Job drawing, mm, ordinate dimensions from the low corner. One solid piece. A direction names the side the tool comes from. Give positions to 0.01 mm unless a question says otherwise; leave off trailing zeros. Loops run counter-clockwise (first coordinate to the right, second up) from the corner with the lowest first, then second, coordinate; pieces in that order, holes last. Notation, with made-up numbers: (-2.5, 62.5) - (10.5, 62.5) arc R24 ccw to (10.5, 93.5) - close; hole circle Ø7 at (-27, 71). An arc over 180 degrees is marked (long way). Use a Markdown table: item, result.
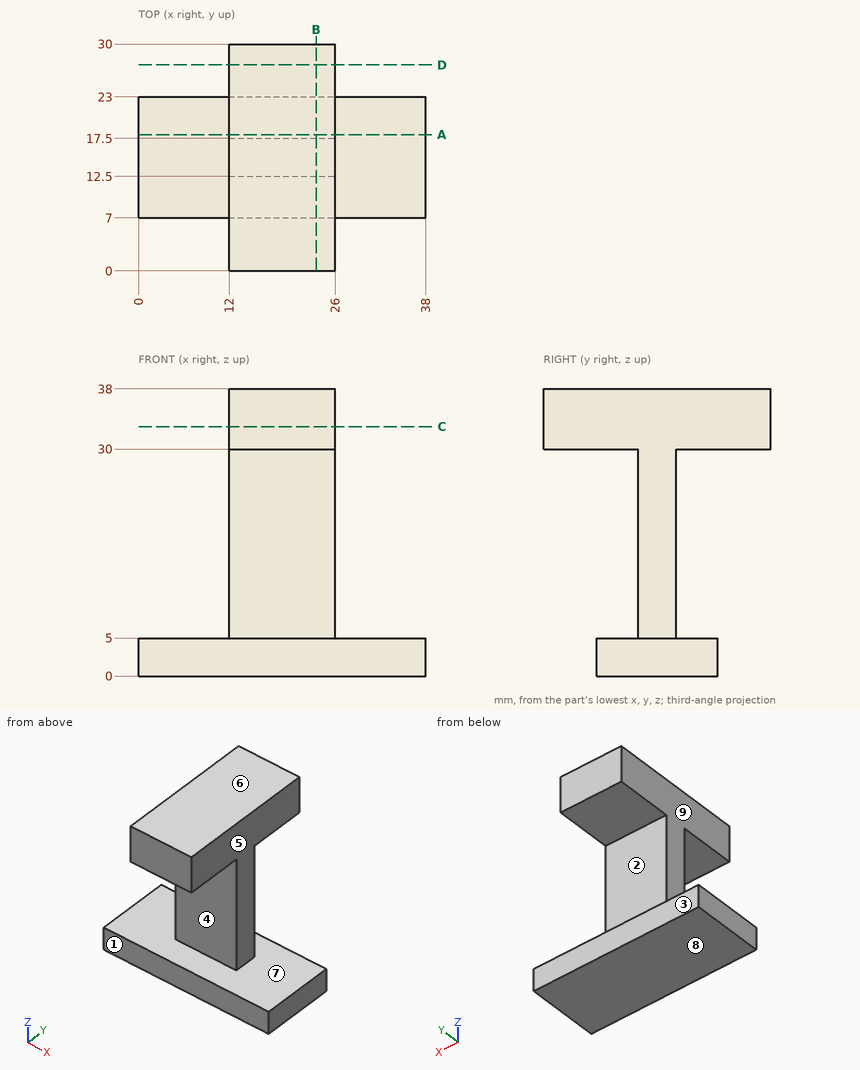
(1) Slice it at B-B, the plane x = 23.5. Write the cut outline in (y, z).
Computed:
| item | result |
|---|---|
| outline | (0, 30) - (12.5, 30) - (12.5, 5) - (7, 5) - (7, 0) - (23, 0) - (23, 5) - (17.5, 5) - (17.5, 30) - (30, 30) - (30, 38) - (0, 38) - close |
(2) Drill centre lines: probe 1 along Z at (x, y) = (7.5, 16.5); probe 2 along Y at (x, z) = (29, 4); probe 3 along Z at (x, y) = (25.5, 2.5). Where is each one in solid material? Low to high. Write a range as [from, to].
Computed:
| item | result |
|---|---|
| probe 1 | [0, 5] |
| probe 2 | [7, 23] |
| probe 3 | [30, 38] |
(3) 3-axis set-ups, long thin cutter, end or side, ignore diameter. For the marked faces 1, 2, 3, 4 and 5: which of +Z, -Z, +X, -X, +Y, -Y reach the whole face in a straight line?
Computed:
| item | result |
|---|---|
| face 1 | -Z, +X, -X, -Y |
| face 2 | +X, -X, +Y |
| face 3 | -Z, +X, -X, +Y |
| face 4 | +X, -X, -Y |
| face 5 | +Z, +X, +Y, -Y |
(4) Slice it at C-C, the plane z = 33. Write the cut outline in (x, y), plus the area to 3 significant figures.
Computed:
| item | result |
|---|---|
| outline | (12, 0) - (26, 0) - (26, 30) - (12, 30) - close |
| area | 420 mm² |
(5) Pin check, flat tips, straight feed: P1, Ø11, axis at x = 20, z = 16.5, coming from the -Y side; P2, Ø1, axis at y = 15, z = 23.5, coming from the +X side; P3, Ø5, axis at y = 23.5, z = 9.5, coming from the +X side; P4, Ø5, axis at y = 25.5, z = 34, coming from the -X side. Stop position of each tip, or through.
Computed:
| item | result |
|---|---|
| P1 | y = 12.5 |
| P2 | x = 26 |
| P3 | through |
| P4 | x = 12 |
(6) Slice it at D-D, the plane y = 27.25. Write the cut outline in (x, z), plus the area to 3 significant figures.
Computed:
| item | result |
|---|---|
| outline | (12, 30) - (26, 30) - (26, 38) - (12, 38) - close |
| area | 112 mm² |
(7) Mould opens along Z. For the marked faces 6, 7, 8 and 9 say: pulls with the +Z half, pulls with the -Z half, needs draft (parallel to the pull), parting line crosses it, or undercut.
Computed:
| item | result |
|---|---|
| face 6 | pulls with the +Z half |
| face 7 | undercut |
| face 8 | pulls with the -Z half |
| face 9 | needs draft |
(8) Slice it at A-A, the plane y = 18. Write the cut outline in (x, z).
Computed:
| item | result |
|---|---|
| outline | (0, 0) - (38, 0) - (38, 5) - (0, 5) - close; (12, 30) - (26, 30) - (26, 38) - (12, 38) - close |
